from build123d import *

# Parameters (mm, degrees)
SKETCH_1_R      = 6
EXTRUDE_1_DEPTH = 6
SKETCH_2_R      = 4
EXTRUDE_2_DEPTH = 120


with BuildPart() as part:
    # 草图1 → 凸台-拉伸1 (new body)
    with BuildSketch(Plane.XY):
        Circle(SKETCH_1_R)
        Polygon((3.464101615, 0), (1.732050808, 3), (-1.732050808, 3), (-3.464101615, 0), (-1.732050808, -3), (1.732050808, -3), align=None, mode=Mode.SUBTRACT)
    extrude(amount=EXTRUDE_1_DEPTH)

    # 草图2 → 凸台-拉伸2 (add)
    with BuildSketch(Plane.XY.offset(6)):
        Circle(SKETCH_2_R)
    extrude(amount=EXTRUDE_2_DEPTH)


solid = part.part
Input: part model. Units: mm. Frame: model coordinates. A direction names the side the tool comes from. Give positions to 0.01 mm unless a question says otherwise; leave off trailing zeros. Order: outer loops, then holes, each group sorted by start corner. A loop starts at its lowest first (then second) coordinate and runs counter-clockwise, first axis right, second up.
Q1. Contact query for flat-ended pins moving along their axis: pin 1 Ø3 at (y, z) = (-5, 110) entering from +X; pin 2 Ø1.5 at (y, z) = (-0.5, 79) entering from -X; pin 3 Ø5 at (y, z) = (4.5, 29.5) entering from -X; pin 4 Ø1 at (x, z) = (0.5, 4) entering from -Y. Output: stop coordinate, or through.
Checked values:
pin 1: stops at x = 1.94
pin 2: stops at x = -4
pin 3: stops at x = -3.46
pin 4: stops at y = -6
Q2. Section A-A on x = 0. Output: boundary loops of the cut face in (y, z).
Checked values:
outline: (-6, 0) - (-3, 0) - (-3, 6) - (3, 6) - (3, 0) - (6, 0) - (6, 6) - (4, 6) - (4, 126) - (-4, 126) - (-4, 6) - (-6, 6) - close
Q3. Section B-B on z = 69. Output: boundary loops of the cut face in (x, y).
Checked values:
outline: circle Ø8 at (0, 0)
Q4. Ray query, probe 1 along Z at (x, y) = (-0.75, -4.5); probe 2 along Y at (x, z) = (-2, 28.5); probe 3 along Z at (x, y) = (0.25, -0.25). Return the intervals inside material, ascending.
Checked values:
probe 1: z = 0 to 6
probe 2: y = -3.46 to 3.46
probe 3: z = 6 to 126
Q5. Draft query along X for faces 1 (the cylindrical face through (-0.867, -3.905, 65.16)), 2 (the flat face through (0, 0, 6)), 3 (the flat face through (-1.42, -3.92, 6)). Return one class per face: +X half, -X half, draft (parallel to the pull), parting line (faces both ways), or undercut.
Checked values:
face 1: parting line
face 2: undercut
face 3: draft
Q6. Set-up query: faces 4 (the flat face through (3, -3, 0)), 5 (the flat face through (0, 3, 3)). Return all of +Z, -Z, +X, -X, +Y, -Y with unobstructed straight access to the full face (end or side cutting, diameter ignored); none if empty.
Checked values:
face 4: -Z, +X, -X, +Y, -Y
face 5: -Z
